```python
from build123d import *

# Parameters (mm, degrees)
SKETCH_1_W      = 36
SKETCH_1_H      = 60
EXTRUDE_1_DEPTH = 2
FILLET_1_R      = 2
SKETCH_2_R      = 1.4
EXTRUDE_2_DEPTH = 2
FILLET_2_R      = 3


with BuildPart() as part:
    # 草图1 → 凸台-拉伸1 (new body)
    with BuildSketch(Plane(origin=(0, 0, 0), x_dir=(1, 0, 0), z_dir=(0, 1, 0))):
        Rectangle(SKETCH_1_W, SKETCH_1_H)
    extrude(amount=EXTRUDE_1_DEPTH)

    # 圆角1
    fillet_1_edges = [part.edges().sort_by_distance(p)[0] for p in [
        (-18, 1, -30),
        (18, 1, -30),
        (18, 1, 30),
        (-18, 1, 30),
    ]]
    fillet(fillet_1_edges, radius=FILLET_1_R)

    # 草图2 → 凸台-拉伸2 (add)
    # profile 1 of 2: a face of its own
    with BuildSketch(Plane(origin=(0, 2, 0), x_dir=(1, 0, 0), z_dir=(0, 1, 0))):
        with BuildLine():
            ThreePointArc((2.236067977, 30), (2.802517077, 30.929533731), (3, 32))
            ThreePointArc((3, 32), (-1.070466269, 34.802517077), (-2.236067977, 30))
            Line((-2.236067977, 30), (2.236067977, 30))
        make_face()
        with Locations(Location((0, 32, 0), (0, 0, 270))):
            Circle(SKETCH_2_R, mode=Mode.SUBTRACT)
    # profile 2 of 2: a face of its own
    with BuildSketch(Plane(origin=(0, 2, 0), x_dir=(1, 0, 0), z_dir=(0, 1, 0))):
        with BuildLine():
            ThreePointArc((-2.236067977, -30), (-1.070466269, -34.802517077), (3, -32))
            ThreePointArc((3, -32), (2.802517077, -30.929533731), (2.236067977, -30))
            Line((2.236067977, -30), (-2.236067977, -30))
        make_face()
        with Locations(Location((0, -32, 0), (0, 0, 270))):
            Circle(SKETCH_2_R, mode=Mode.SUBTRACT)
    extrude(amount=-EXTRUDE_2_DEPTH)

    # 圆角2
    fillet_2_edges = [part.edges().sort_by_distance(p)[0] for p in [
        (2.236067977, 1, -30),
        (-2.236067977, 1, -30),
        (2.236067977, 1, 30),
        (-2.236067977, 1, 30),
    ]]
    fillet(fillet_2_edges, radius=FILLET_2_R)


solid = part.part
```
Geometry check sheet. Reference: the model listing, model coordinates, mm. A direction names the side the tool comes from. Round coordinates to 2 decimals unless told otherwise and drop trailing zeros. Loops run counter-clockwise (first coordinate to the right, second up) from the corner with the lowest first, then second, coordinate; pieces in that order, holes last. Notation, with made-up numbers: (50.5, 24) -> (85.5, 24) arc R24 ccw to (85.5, 39) -> close; hole circle Ø5 at (56, -36). An arc over 180 degrees is marked (long way). Use a Markdown table: item, result.
(1) Go/stop test with flat-tipped pins: P1, Ø0.6, axis at x = 12.5, y = 1, coming from the +Z side; P2, Ø1, axis at x = -1, y = 1, coming from the +Z side. Record where each tip stops, or that it passes through.
Calculated:
| item | result |
|---|---|
| P1 | z = 30 |
| P2 | z = 34.96 |
(2) Mould release check, pull along X, two halves, no side actions. Record for faces 1 (the flat face through (11, 1, 30)), 2 (the cylindrical face through (-17.43, 1.01, -29.4)), 3 (the cylindrical face through (0.06, 1.01, 30.6)): released by +X, released by -X, zero draft, split by the parting line, or undercut.
Calculated:
| item | result |
|---|---|
| face 1 | zero draft |
| face 2 | released by -X |
| face 3 | undercut |
(3) Sectioned sample at A-A (x = 0). Enter the section's corners in (y, z).
Calculated:
| item | result |
|---|---|
| outline | (0, -35) -> (2, -35) -> (2, -33.4) -> (0, -33.4) -> close; (0, -30.6) -> (2, -30.6) -> (2, 30.6) -> (0, 30.6) -> close; (0, 33.4) -> (2, 33.4) -> (2, 35) -> (0, 35) -> close |
(4) Sectioned sample at B-B (x = -11). Enter the section's corners in (y, z), then the cut area to 3 significant figures.
Calculated:
| item | result |
|---|---|
| outline | (0, -30) -> (2, -30) -> (2, 30) -> (0, 30) -> close |
| area | 120 mm² |
(5) Scan lines: probe 1 along Z at (x, y) = (-0.5, 0.1); probe 2 along Z at (x, y) = (14, 1.45); probe 3 along X at (y, z) = (0.85, -32). Record each from-to range of solid material in increasing order.
Calculated:
| item | result |
|---|---|
| probe 1 | -34.96 to -33.31, -30.69 to 30.69, 33.31 to 34.96 |
| probe 2 | -30 to 30 |
| probe 3 | -3.09 to -1.4, 1.4 to 3.09 |
(6) Set-up check for faces 4 (the flat face through (-11, 1, -30)), 5 (the flat face through (-11, 1, 30)), 6 (the flat face through (11, 1, -30)): record each of +Z, -Z, +X, -X, +Y, -Y from which the full face is reachable in a straight line by a thin tool's end or side.
Calculated:
| item | result |
|---|---|
| face 4 | -Z, -X, +Y, -Y |
| face 5 | +Z, -X, +Y, -Y |
| face 6 | -Z, +X, +Y, -Y |
